For this review, take the finished solid that the model builds, in its own axes (mm). A direction names the side the tool comes from. Coordinates: 2 decimals unless noted, no trailing zeros. Loops run counter-clockwise (first coordinate to the right, second up) from the corner with the lowest first, then second, coordinate; pieces in that order, holes last. Notation, with made-up numbers: (75, 33.5) -> (119, 33.5) arc R13 ccw to (119, 51.5) -> close; hole circle Ø6 at (68, 36.25). An arc over 180 degrees is marked (long way). Answer in a Markdown table with one row per item.
Autodesk Inventor part; units mm, degrees
ref_plane "YZ Plane" through (0, 0, 0) normal (1, 0, 0) x (0, 1, 0)
ref_plane "XZ Plane" through (0, 0, 0) normal (0, 1, 0) x (-1, 0, 0)
ref_plane "XY Plane" through (0, 0, 0) normal (0, 0, 1) x (1, 0, 0)
sketch "Sketch1" plane through (0, 0, 0) normal (0, 0, 1) x (1, 0, 0)
  line L0 (0, 0) -> (70, 0)
  line L1 (70, 0) -> (70, -200)
  line L2 (70, -200) -> (0, -200)
  line L3 (0, -200) -> (0, 0)
  dimension "d0" = 70
  dimension "d1" = 200
extrude "Extrusion1" add sketch "Sketch1" along normal blind 5
sketch "Sketch3" plane through (0, 0, 5) normal (0, 0, 1) x (1, 0, 0)
  line L0 (0, -0.5) -> (0, -3)
  line L1 (0, -3) -> (0, -30)
  line L2 (0, -3) -> (0, -2)
  line L3 (8, -1) -> (11, -1)
  line L4 (0, -30) -> (0, -28.5)
  line L5 (8, -28.5) -> (8, -26.5)
  line L6 (13, -26.5) -> (13, -33.5)
  line L7 (8, -33.5) -> (8, -31.5)
  line L8 (0, -31.5) -> (0, -30)
  line L9 (0, -30) -> (13, -30)
  line L10 (0, -30) -> (0, -60)
  line L11 (0, -60) -> (13, -60)
  line L12 (13, -60) -> (13, -56.5)
  line L13 (13, -56.5) -> (8, -56.5)
  line L14 (8, -56.5) -> (8, -58.5)
  line L15 (8, -58.5) -> (0, -58.5)
  line L16 (13, -60) -> (13, -63.5)
  line L17 (13, -63.5) -> (8, -63.5)
  line L18 (8, -63.5) -> (8, -61.5)
  line L19 (8, -61.5) -> (0, -61.5)
  line L20 (0, -60) -> (0, -90)
  line L21 (0, -90) -> (0, -170)
  line L22 (0, -170) -> (13, -170)
  line L23 (13, -170) -> (13, -166.5)
  line L24 (13, -166.5) -> (8, -166.5)
  line L25 (8, -166.5) -> (8, -168.5)
  line L26 (8, -168.5) -> (0, -168.5)
  line L27 (13, -170) -> (13, -173.5)
  line L28 (13, -173.5) -> (8, -173.5)
  line L29 (8, -173.5) -> (8, -171.5)
  line L30 (8, -171.5) -> (0, -171.5)
  line L31 (0, -171.5) -> (0, -170)
  line L32 (0, -91.5) -> (0, -90)
  line L33 (0, -61.5) -> (0, -60)
  line L34 (0, -31.5) -> (0, -30)
  line L35 (0, -4) -> (0, -3)
  line L36 (70, 0) -> (0, 0)
  line L37 (0, -30) -> (70, -30)
  line L38 (0, -60) -> (70, -60)
  line L39 (0, -170) -> (70, -170)
  line L40 (70, -60) -> (70, -58.5)
  line L41 (70, -58.5) -> (62, -58.5)
  line L42 (62, -58.5) -> (62, -56.5)
  line L43 (62, -56.5) -> (57, -56.5)
  line L44 (57, -56.5) -> (57, -60)
  line L45 (57, -60) -> (57, -63.5)
  line L46 (57, -63.5) -> (62, -63.5)
  line L47 (62, -63.5) -> (62, -61.5)
  line L48 (62, -61.5) -> (70, -61.5)
  line L49 (70, -61.5) -> (70, -60)
  line L50 (70, -170) -> (70, -168.5)
  line L51 (70, -168.5) -> (62, -168.5)
  line L52 (62, -168.5) -> (62, -166.5)
  line L53 (62, -166.5) -> (57, -166.5)
  line L54 (57, -166.5) -> (57, -170)
  line L55 (70, -170) -> (70, -171.5)
  line L56 (70, -171.5) -> (62, -171.5)
  line L57 (62, -171.5) -> (62, -173.5)
  line L58 (62, -173.5) -> (57, -173.5)
  line L59 (57, -173.5) -> (57, -170)
  line L60 (13, -33.5) -> (8, -33.5)
  line L61 (13, -26.5) -> (8, -26.5)
  line L62 (8, -28.5) -> (0, -28.5)
  line L63 (8, -31.5) -> (0, -31.5)
  line L64 (70, -28.5) -> (62, -28.5)
  line L65 (62, -28.5) -> (62, -26.5)
  line L66 (62, -26.5) -> (57, -26.5)
  line L67 (57, -26.5) -> (57, -30)
  line L68 (57, -30) -> (57, -33.5)
  line L69 (57, -33.5) -> (62, -33.5)
  line L70 (62, -33.5) -> (62, -31.5)
  line L71 (62, -31.5) -> (70, -31.5)
  line L72 (70, -28.5) -> (70, -30)
  line L73 (70, -30) -> (70, -31.5)
  line L74 (0, -0.5) -> (0, 0)
  dimension "d35" = 3
  dimension "d41" = 5
  dimension "d53" = 2
  dimension "d55" = 5
  dimension "d92" = 1.5
  dimension "d94" = 1.5
  dimension "d95" = 2
  dimension "d97" = 8
  dimension "d99" = 5
  dimension "d103" = 1.5
  dimension "d104" = 1.5
  dimension "d105" = 8
  dimension "d113" = 1.5
  dimension "d114" = 1.5
  dimension "d115" = 8
  dimension "d116" = 5
  dimension "d117" = 2
  dimension "d118" = 2
  dimension "d130" = 1.5
  dimension "d131" = 8
  dimension "d132" = 2
  dimension "d133" = 5
  dimension "d134" = 3.5
  dimension "d135" = 5
  dimension "d136" = 2
  dimension "d145" = 1.5
  dimension "d146" = 8
  dimension "d147" = 2
  dimension "d148" = 5
  dimension "d149" = 1.5
  dimension "d150" = 8
  dimension "d151" = 2
  dimension "d152" = 5
extrude "Extrusion3" cut sketch "Sketch3" against normal blind 5 contours L22 L27 L28 L29 L30 L31
extrude "Extrusion4" cut sketch "Sketch3" against normal blind 5 contours L26 L25 L24 L23 L22 L21
extrude "Extrusion14" cut sketch "Sketch3" against normal blind 5 contours L39 L55 L56 L57 L58 L59
extrude "Extrusion15" cut sketch "Sketch3" against normal blind 5 contours L54 L53 L52 L51 L50 L39
sketch "Sketch4" plane through (0, 0, 5) normal (0, 0, 1) x (1, 0, 0)
  line L0 (0, 0) -> (0, -19)
  circle A0 centre (11.4, -69) radius 6
  line L1 (17.4, -69) -> (34.103, -69)
  circle A1 centre (35.353, -69) radius 1.25
  line L2 (35.353, -69) -> (34.103, -69)
  line L3 (35.353, -69) -> (32.177, -69)
  line L4 (32.177, -69) -> (32.177, -78.842)
  line L5 (32.177, -69) -> (32.177, -59.158)
  circle A2 centre (32.177, -59.158) radius 1.25
  circle A3 centre (32.177, -78.842) radius 1.25
  line L6 (35.353, -69) -> (18.403, -69)
  line L7 (18.403, -69) -> (18.403, -85.95)
  line L8 (18.403, -69) -> (18.403, -52.05)
  circle A4 centre (18.403, -52.05) radius 1.25
  circle A5 centre (18.403, -85.95) radius 1.25
  line L9 (32.177, -59.158) -> (18.403, -52.05)
  line L10 (18.403, -69) -> (17.4, -69)
  line L11 (18.403, -69) -> (4.629, -69)
  line L12 (18.403, -52.05) -> (4.629, -59.158)
  circle A6 centre (4.629, -59.158) radius 1.25
  line L13 (4.629, -59.158) -> (4.629, -78.842)
  line L14 (18.403, -85.95) -> (4.629, -78.842)
  circle A7 centre (4.629, -78.842) radius 1.25
  line L15 (70, 0) -> (0, 0)
  dimension "d171" = 12
  dimension "d176" = 2.5
  dimension "d169" = 19
  dimension "d179" = 3.176
  dimension "d180" = 9.842
  dimension "d181" = 9.842
  dimension "d182" = 2.5
  dimension "d183" = 2.5
  dimension "d184" = 16.95
  dimension "d185" = 16.95
  dimension "d186" = 16.95
  dimension "d187" = 2.5
  dimension "d188" = 2.5
  dimension "d196" = 13.774
  dimension "d197" = 2.5
  dimension "d273" = 69
extrude "Extrusion22" cut sketch "Sketch4" against normal blind 5 contours L11 A0 | A0 L11
hole "Hole1" at (18.403, -85.95, 5) direction (0, 0, -1) diameter 2.5 end through all
hole "Hole2" at (4.629, -78.842, 5) at (4.629, -59.158, 5) at (4.629, -78.842, 5) direction (0, 0, -1) diameter 2.5 end through all
hole "Hole3" at (18.403, -52.05, 5) direction (0, 0, -1) diameter 2.5 end through all
hole "Hole4" at (32.177, -59.158, 5) direction (0, 0, -1) diameter 2.5 end through all
hole "Hole5" at (35.353, -69, 5) direction (0, 0, -1) diameter 2.5 end through all
hole "Hole6" at (32.177, -78.842, 5) direction (0, 0, -1) diameter 2.5 end through all
sketch "Sketch5" plane through (70, -200, 5) normal (1, 0, 0) x (0, 0, -1)
  line L0 (0, 0) -> (0, 15)
  line L1 (0, 15) -> (5, 15)
  line L2 (5, 15) -> (5, 25)
  line L3 (5, 25) -> (0, 25)
  line L4 (0, 25) -> (0, 15)
  line L5 (0, 25) -> (0, 35)
  line L6 (0, 35) -> (5, 35)
  line L7 (5, 35) -> (5, 45)
  line L8 (5, 45) -> (0, 45)
  line L9 (0, 45) -> (0, 35)
  line L10 (5, 200) -> (0, 200)
  line L11 (0, 185) -> (5, 185)
  line L12 (5, 185) -> (5, 175)
  line L13 (5, 175) -> (0, 175)
  line L14 (0, 175) -> (0, 185)
  line L15 (0, 175) -> (0, 165)
  line L16 (0, 165) -> (5, 165)
  line L17 (5, 165) -> (5, 155)
  line L18 (5, 155) -> (0, 155)
  line L19 (0, 155) -> (0, 165)
  dimension "d242" = 15
  dimension "d243" = 10
  dimension "d244" = 10
  dimension "d245" = 10
  dimension "d247" = 10
  dimension "d248" = 10
  dimension "d249" = 10
  dimension "d269" = 110
extrude "Extrusion26" add sketch "Sketch5" along normal blind 5
sketch "Sketch6" plane through (0, 0, 0) normal (-1, 0, 0) x (0, 0, 1)
  line L0 (0, 0) -> (0, -15)
  line L1 (0, -15) -> (0, -25)
  line L2 (0, -25) -> (5, -25)
  line L3 (5, -25) -> (5, -15)
  line L4 (5, -15) -> (0, -15)
  line L5 (0, -25) -> (0, -35)
  line L6 (0, -35) -> (5, -35)
  line L7 (5, -35) -> (5, -45)
  line L8 (5, -45) -> (0, -45)
  line L9 (0, -45) -> (0, -35)
  line L10 (5, -45) -> (5, -150)
  line L11 (5, -150) -> (5, -185)
  line L12 (0, -185) -> (0, -175)
  line L13 (0, -175) -> (0, -165)
  line L14 (0, -165) -> (5, -165)
  line L15 (5, -165) -> (5, -155)
  line L16 (5, -155) -> (0, -155)
  line L17 (0, -155) -> (0, -165)
  line L18 (5, -155) -> (5, -45)
  line L19 (0, -185) -> (5, -185)
  line L20 (0, -175) -> (5, -175)
  dimension "d253" = 10
  dimension "d254" = 5
  dimension "d255" = 10
  dimension "d256" = 10
  dimension "d259" = 10
  dimension "d260" = 10
  dimension "d261" = 10
  dimension "d266" = 110
extrude "Extrusion28" add sketch "Sketch6" along normal blind 5 contours L4 L3 L2 L1 | L11 L14 L17 L16 | L6 L7 L8 L9 | L11 L19 L12 L20
extrude "Extrusion30" cut sketch "Sketch3" against normal blind 5 contours L62 L5 L61 L6 L9 L1 | L67 L66 L65 L64 L72 L37 | L37 L73 L71 L70 L69 L68 | L9 L6 L60 L7 L63 L8
properties part number "lateral_mdf"
Item 1: For faces 1 (the flat face through (11, -33.5, 3)), 2 (the flat face through (-2, -15, 3)), 3 (the flat face through (66, -171.5, 3)), 4 (the flat face through (4, -168.5, 3)), list the 3-axis set-ups (+Z, -Z, +X, -X, +Y, -Y) from which the entire face can be reached by the end or side of a thin tool; tool diameter is ignored.
Worked answers:
| item | result |
|---|---|
| face 1 | +Z, -Z |
| face 2 | +Z, -Z, -X, +Y |
| face 3 | +Z, -Z, +X |
| face 4 | +Z, -Z, -X |
Item 2: Take a section at B-B, the plane y = -66. State the section outline as (x, z) points.
Worked answers:
| item | result |
|---|---|
| outline | (0, 0) -> (6.2, 0) -> (6.2, 5) -> (0, 5) -> close; (16.6, 0) -> (70, 0) -> (70, 5) -> (16.6, 5) -> close |
Item 3: Insertion check: pin 1 (1.6 mm diameter, centred on y = -168, z = 2.5, fed in from -X); pin 2 (2 mm diameter, centred on y = -142, z = 1.5, fed in from +X). Each pin has a flat end and moves straight along its axis. Give the tip position at first contact, or say it passes through.
Worked answers:
| item | result |
|---|---|
| pin 1 | x = 0 |
| pin 2 | x = 70 |
Item 4: Take a section at A-A, the plane x = 65. State the section outline as (y, z) points, and give its area (3 significant figures).
Worked answers:
| item | result |
|---|---|
| outline | (-200, 0) -> (-171.5, 0) -> (-171.5, 5) -> (-200, 5) -> close; (-168.5, 0) -> (-31.5, 0) -> (-31.5, 5) -> (-168.5, 5) -> close; (-28.5, 0) -> (0, 0) -> (0, 5) -> (-28.5, 5) -> close |
| area | 970 mm² |
Item 5: Take a section at C-C, the plane y = -126. State the section outline as (x, z) points.
Worked answers:
| item | result |
|---|---|
| outline | (0, 0) -> (70, 0) -> (70, 5) -> (0, 5) -> close |
Item 6: Take a section at D-D, the plane z = 1.7. Count the separate pieces of the cut face and the enclosed holes in it, and give its area (3 significant figures).
Worked answers:
| item | result |
|---|---|
| separate pieces | 1 |
| enclosed holes | 8 |
| area | 14,000 mm² |
Item 7: The part is to be moulded in two halves that separate along Y. For faces 5 (the flat face through (0, -167, 2)), 6 (the flat face through (70, -27, 2)), 7 (the flat face through (35, 0, 2)), 8 (the flat face through (-5, -20, 2)), say which applies: +Y half, -Y half, draft (parallel to the pull), parting line (faces both ways), or undercut.
Worked answers:
| item | result |
|---|---|
| face 5 | undercut |
| face 6 | undercut |
| face 7 | +Y half |
| face 8 | draft |
Item 8: For L1, parallel to Y at x = 4.5, z = 1.3; L2, parallel to Y at x = 11.4, z = 3.8; L3, parallel to X at y = -59, z = 3.85, list the stretches that pass through material, from the lowest coordinate up.
Worked answers:
| item | result |
|---|---|
| L1 | -200 to -171.5, -168.5 to -80.09, -77.6 to -60.4, -57.91 to -31.5, -28.5 to 0 |
| L2 | -200 to -173.5, -166.5 to -75, -63 to -33.5, -26.5 to 0 |
| L3 | 0 to 3.39, 5.87 to 30.94, 33.42 to 70 |
